Could you check a few things on this model? Use its own coordinates, in mm. A direction names the side the tool comes from. Give positions to 0.01 mm unless a question says otherwise; leave off trailing zeros. Order: outer loops, then holes, each group sorted by start corner. A loop starts at its lowest first (then second) coordinate and runs counter-clockwise, first axis right, second up.
(1) Will these pins go through, and if not, where does the flat tip stop? pin 1 (0.5 mm diameter, centred on x = 18.5, y = 17.5, fed in from +Z); pin 2 (2 mm diameter, centred on x = 15.5, y = 18.5, fed in from -Z); pin 3 (3.5 mm diameter, centred on y = 17.5, z = 23.5, fed in from -X); pin 4 (2 mm diameter, centred on x = 15, y = 17.725, fed in from +Z).
(2) Imagine slicing it at B-B, the plane z = 19.5. State how many separate pieces and enclosed holes the cut face has, then the cut area to 3 significant figures.
(3) Imagine slicing it at C-C, the plane x = 15. Write out the boundary of the cut face in (y, z) (3 decimals).
(4) If I drill on probe 1 along X at (y, z) = (13.75, 16.25); probe 2 along X at (y, z) = (17.5, 16.5); probe 3 along X at (y, z) = (11.75, 15.5) (3 decimals), over which ranges is the centre line in solid material (lowest first)?
(5) On a 3-axis mill with a long thin cutter (end or side, diameter ignored), from which of +Z, -Z, +X, -X, +Y, -Y can I reach the whole of each face in a straight line? I mean faces 4 (the flat face through (9.85, 18, 23)), 5 (the flat face through (-0.056, 12.391, 16.951)), 6 (the cylindrical face through (2.2, 16.95, 16.95)), 7 (the flat face through (-4, 10.85, 17)). Say none if no direction works.
(6) If we mould it in two halves opening along X, with no side actions, what happens to faces 1 (the flat face through (4.657, 12.391, 16.951)), 2 (the flat face through (-13, 10.85, 17)), 3 (the flat face through (7.14, 12.43, 16.95))? For each: released by +X, released by -X, zero draft, split by the parting line, or undercut.
(7) Imagine slicing it at A-A, the plane y = 12.5. Write out the boundary of the cut face in (x, z).
(8) Imagine slicing it at D-D, the plane y = 19. Write out the boundary of the cut face in (x, z).
from build123d import *

# Parameters (mm, degrees)
BOSS_EXTRUDE1_START     = 13.5
BOSS_EXTRUDE1_DEPTH     = 7
BOSS_EXTRUDE2_START     = 14
SKETCH2_W               = 13
SKETCH2_H               = 4.5
BOSS_EXTRUDE2_DEPTH     = 11
CUT_EXTRUDE1_START      = 21.7
SKETCH3_W               = 3.3
SKETCH3_H               = 4.2
CUT_EXTRUDE1_DEPTH      = 3.4
CUT_EXTRUDE2_START      = 16
SKETCH4_R               = 0.9
CUT_EXTRUDE2_DEPTH      = 9.1
CUT_EXTRUDE3_DEPTH      = 40.40812892
CUT_EXTRUDE3_DEPTH_BACK = 40.40812892
SKETCH5_W               = 19
SKETCH5_H               = 2.4
CUT_EXTRUDE4_DEPTH      = 40.40812892
CUT_EXTRUDE4_DEPTH_BACK = 40.40812892
SKETCH6_R               = 1.2


with BuildPart() as part:
    # Sketch1 → Boss-Extrude1 (new body)
    with BuildSketch(Plane.XY.offset(BOSS_EXTRUDE1_START)):
        Polygon((-23, 19.975), (13, 19.975), (13, 13.975), (7.70102766, 13.975), (6.563620678, 10.85), (5.217351773, 10.85), (4.079944791, 13.975), (2.988638679, 13.975), (1.851231697, 10.85), (0.504962793, 10.85), (-0.632444189, 13.975), (-1.723750301, 13.975), (-2.861157283, 10.85), (-4.207426188, 10.85), (-5.34483317, 13.975), (-6.436139281, 13.975), (-7.573546263, 10.85), (-8.919815168, 10.85), (-10.05722215, 13.975), (-11.148528262, 13.975), (-12.285935244, 10.85), (-13.632204148, 10.85), (-14.76961113, 13.975), (-23, 13.975), align=None)
    extrude(amount=BOSS_EXTRUDE1_DEPTH)

    # Sketch2 → Boss-Extrude2 (add)
    with BuildSketch(Plane.XY.offset(BOSS_EXTRUDE2_START)):
        with Locations((14.5, 17.725)):
            Rectangle(SKETCH2_W, SKETCH2_H)
    extrude(amount=BOSS_EXTRUDE2_DEPTH)

    # Sketch3 → Cut-Extrude1 (cut)
    with BuildSketch(Plane.XY.offset(CUT_EXTRUDE1_START)):
        with Locations((11.5, 17.725)):
            Rectangle(SKETCH3_W, SKETCH3_H)
    extrude(amount=CUT_EXTRUDE1_DEPTH, mode=Mode.SUBTRACT)

    # Sketch4 → Cut-Extrude2 (cut)
    with BuildSketch(Plane.XY.offset(CUT_EXTRUDE2_START)):
        with Locations((15, 17.725)):
            Circle(SKETCH4_R)
        with Locations((18.5, 17.725)):
            Circle(SKETCH4_R)
    extrude(amount=CUT_EXTRUDE2_DEPTH, mode=Mode.SUBTRACT)

    # Sketch5 → Cut-Extrude3 (cut, two sides: drawn at the far end of the back side and taken through both)
    with BuildSketch(Plane.XY.offset(-CUT_EXTRUDE3_DEPTH_BACK)):
        with Locations((-8.5, 16.975)):
            Rectangle(SKETCH5_W, SKETCH5_H)
    extrude(amount=CUT_EXTRUDE3_DEPTH + CUT_EXTRUDE3_DEPTH_BACK, mode=Mode.SUBTRACT)

    # Sketch6 → Cut-Extrude4 (cut, two sides: drawn at the far end of the back side and taken through both)
    with BuildSketch(Plane.XY.offset(-CUT_EXTRUDE4_DEPTH_BACK)):
        with Locations((-18, 16.975)):
            Circle(SKETCH6_R)
        with Locations((1, 16.975)):
            Circle(SKETCH6_R)
    extrude(amount=CUT_EXTRUDE4_DEPTH + CUT_EXTRUDE4_DEPTH_BACK, mode=Mode.SUBTRACT)


solid = part.part
Answer block:
1. pin 1: stops at z = 16
1. pin 2: stops at z = 14
1. pin 3: stops at x = 8
1. pin 4: stops at z = 25
2. separate pieces: 1
2. enclosed holes: 3
2. area: 236 mm2
3. outline: (15.475, 14) - (19.975, 14) - (19.975, 25) - (18.625, 25) - (18.625, 16) - (16.825, 16) - (16.825, 25) - (15.475, 25) - close
4. probe 1: x = -14.69 to -11.23, -9.98 to -6.52, -5.26 to -1.81, -0.55 to 2.91, 4.16 to 7.62
4. probe 2: x = -23 to -19.08, 2.08 to 14.13, 15.87 to 17.63, 19.37 to 21
4. probe 3: x = -13.96 to -11.958, -9.247 to -7.246, -4.535 to -2.534, 0.177 to 2.179, 4.89 to 6.891
5. face 4: +Z
5. face 5: +Z, -Z, -Y
5. face 6: +Z, -Z
5. face 7: +Z, -Z, +X, -X, -Y
6. face 1: undercut
6. face 2: zero draft
6. face 3: released by +X
7. outline: (-14.23, 13.5) - (-11.69, 13.5) - (-11.69, 20.5) - (-14.23, 20.5) - close; (-9.52, 13.5) - (-6.97, 13.5) - (-6.97, 20.5) - (-9.52, 20.5) - close; (-4.81, 13.5) - (-2.26, 13.5) - (-2.26, 20.5) - (-4.81, 20.5) - close; (-0.1, 13.5) - (2.45, 13.5) - (2.45, 20.5) - (-0.1, 20.5) - close; (4.62, 13.5) - (7.16, 13.5) - (7.16, 20.5) - (4.62, 20.5) - close
8. outline: (-23, 13.5) - (13, 13.5) - (13, 14) - (21, 14) - (21, 25) - (13.15, 25) - (13.15, 21.7) - (9.85, 21.7) - (9.85, 25) - (8, 25) - (8, 20.5) - (-23, 20.5) - close
